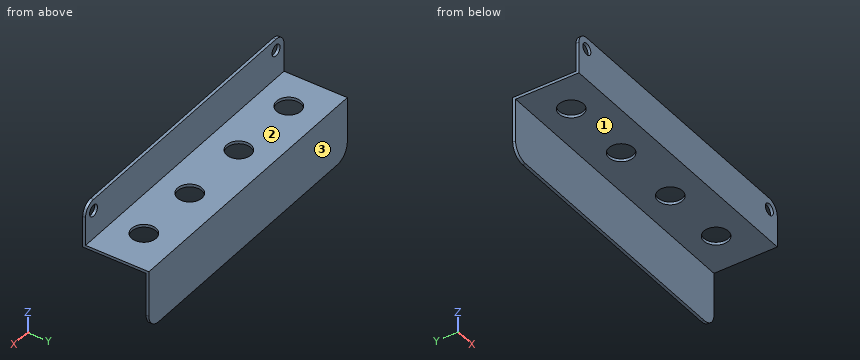
from build123d import *

# Parameters (mm, degrees)
SKETCH1_W           = 100
SKETCH1_H           = 20
BOSS_EXTRUDE1_DEPTH = 1
SKETCH3_W           = 100
SKETCH3_H           = 23
BOSS_EXTRUDE2_DEPTH = 1
SKETCH4_W           = 100
SKETCH4_H           = 14
SKETCH4_R           = 2
BOSS_EXTRUDE3_DEPTH = 1
FILLET1_R           = 4
CUT_EXTRUDE2_REACH  = 60.523
SKETCH6_R           = 4.25
FILLET2_R           = 5


with BuildPart() as part:
    # Sketch1 → Boss-Extrude1 (new body)
    with BuildSketch(Plane(origin=(0, 0, 0), x_dir=(1, 0, 0), z_dir=(0, 1, 0))):
        Rectangle(SKETCH1_W, SKETCH1_H)
    extrude(amount=BOSS_EXTRUDE1_DEPTH)

    # Sketch3 → Boss-Extrude2 (add)
    with BuildSketch(Plane.XY.offset(10)):
        with Locations((0, -10.5)):
            Rectangle(SKETCH3_W, SKETCH3_H)
    extrude(amount=BOSS_EXTRUDE2_DEPTH)

    # Sketch4 → Boss-Extrude3 (add)
    with BuildSketch(Plane.XZ.offset(22)):
        with Locations((0, 18)):
            Rectangle(SKETCH4_W, SKETCH4_H)
        with Locations(Location((46, 21, 0), (0, 0, 270))):
            Circle(SKETCH4_R, mode=Mode.SUBTRACT)
        with Locations(Location((-46, 21, 0), (0, 0, 270))):
            Circle(SKETCH4_R, mode=Mode.SUBTRACT)
    extrude(amount=-BOSS_EXTRUDE3_DEPTH)

    # Fillet1
    fillet1_edges = [part.edges().sort_by_distance(p)[0] for p in [
        (-50, -21.5, 25),
        (50, -21.5, 25),
    ]]
    fillet(fillet1_edges, radius=FILLET1_R)

    # Sketch6 → Cut-Extrude2 (cut, up to next)
    with BuildSketch(Plane.XY.offset(11), mode=Mode.PRIVATE) as cut_extrude2_sk1:
        with Locations((-37.172974346, -10.5)):
            Circle(SKETCH6_R)
    cut_extrude2_tool1 = extrude(cut_extrude2_sk1.sketch, amount=-CUT_EXTRUDE2_REACH, mode=Mode.PRIVATE) & part.part
    # Sketch6 → Cut-Extrude2 (cut, up to next)
    with BuildSketch(Plane.XY.offset(11), mode=Mode.PRIVATE) as cut_extrude2_sk2:
        with Locations((-12.026924054, -10.5)):
            Circle(SKETCH6_R)
    cut_extrude2_tool2 = extrude(cut_extrude2_sk2.sketch, amount=-CUT_EXTRUDE2_REACH, mode=Mode.PRIVATE) & part.part
    # Sketch6 → Cut-Extrude2 (cut, up to next)
    with BuildSketch(Plane.XY.offset(11), mode=Mode.PRIVATE) as cut_extrude2_sk3:
        with Locations((12.738125476, -10.5)):
            Circle(SKETCH6_R)
    cut_extrude2_tool3 = extrude(cut_extrude2_sk3.sketch, amount=-CUT_EXTRUDE2_REACH, mode=Mode.PRIVATE) & part.part
    # Sketch6 → Cut-Extrude2 (cut, up to next)
    with BuildSketch(Plane.XY.offset(11), mode=Mode.PRIVATE) as cut_extrude2_sk4:
        with Locations((35.852171704, -10.5)):
            Circle(SKETCH6_R)
    cut_extrude2_tool4 = extrude(cut_extrude2_sk4.sketch, amount=-CUT_EXTRUDE2_REACH, mode=Mode.PRIVATE) & part.part
    add(cut_extrude2_tool1.solids().sort_by_distance((-37.172974, -10.5, 11))[0], mode=Mode.SUBTRACT)
    add(cut_extrude2_tool2.solids().sort_by_distance((-12.026924, -10.5, 11))[0], mode=Mode.SUBTRACT)
    add(cut_extrude2_tool3.solids().sort_by_distance((12.738125, -10.5, 11))[0], mode=Mode.SUBTRACT)
    add(cut_extrude2_tool4.solids().sort_by_distance((35.852172, -10.5, 11))[0], mode=Mode.SUBTRACT)

    # Fillet2
    fillet2_edges = [part.edges().sort_by_distance(p)[0] for p in [
        (-50, 0.5, -10),
        (50, 0.5, -10),
    ]]
    fillet(fillet2_edges, radius=FILLET2_R)


solid = part.part
Verification items for the finished model (mm, model axes). Face numbers are marked on the shaded views. A direction names the side the tool comes from. Coordinates: 2 decimals unless noted, no trailing zeros. Order: outer loops, then holes, each group sorted by start corner. A loop starts at its lowest first (then second) coordinate and runs counter-clockwise, first axis right, second up.
Item 1: Material ranges on L1, parallel to Y at x = 18, z = -1; L2, parallel to Z at x = 4.5, y = -2.75; L3, parallel to Y at x = 33, z = 18, recorded low to high.
Filled in:
L1: y = 0 to 1
L2: z = 10 to 11
L3: y = -22 to -21
Item 2: Depth check by flat-ended pin: pin 1 (4 mm diameter, centred on x = 30, y = -10.5, fed in from -Z); pin 2 (6.5 mm diameter, centred on x = -46, z = 21, fed in from +Y); pin 3 (6.5 mm diameter, centred on x = -1.5, y = -11, fed in from +Z). Enter the tip coordinate at first touch or a pass-through.
Filled in:
pin 1: stops at z = 10
pin 2: stops at y = -21
pin 3: stops at z = 11
Item 3: Access from +Z, -Z, +X, -X, +Y, -Y to the whole of each face (thin tool, end or side, straight path). Record for the marked faces 1, 2 and 3.
Filled in:
face 1: -Z, +X, -X, -Y
face 2: +Z, +X, -X, +Y
face 3: +Z, -Z, +X, -X, +Y
Item 4: Section check D-D, the plane y = -5. Enter the section's corners in (x, z).
Filled in:
outline: (-50, 10) - (50, 10) - (50, 11) - (-50, 11) - close
Item 5: Section check C-C, the plane x = -14. Enter the section's corners in (y, z), then the cut area to 3 significant figures.
Filled in:
outline: (-22, 10) - (-14.26, 10) - (-14.26, 11) - (-21, 11) - (-21, 25) - (-22, 25) - close; (-6.74, 10) - (0, 10) - (0, -10) - (1, -10) - (1, 11) - (-6.74, 11) - close
area: 49.5 mm2
Item 6: Section check A-A, the plane y = -10.5. Enter the section's corners in (x, z), then the cut area to 3 significant figures.
Filled in:
outline: (-50, 10) - (-41.42, 10) - (-41.42, 11) - (-50, 11) - close; (-32.92, 10) - (-16.28, 10) - (-16.28, 11) - (-32.92, 11) - close; (-7.78, 10) - (8.49, 10) - (8.49, 11) - (-7.78, 11) - close; (16.99, 10) - (31.6, 10) - (31.6, 11) - (16.99, 11) - close; (40.1, 10) - (50, 10) - (50, 11) - (40.1, 11) - close
area: 66.0 mm2
Item 7: Section check B-B, the plane x = -24. Enter the section's corners in (y, z), then the cut area to 3 significant figures.
Filled in:
outline: (-22, 10) - (0, 10) - (0, -10) - (1, -10) - (1, 11) - (-21, 11) - (-21, 25) - (-22, 25) - close
area: 57.0 mm2
